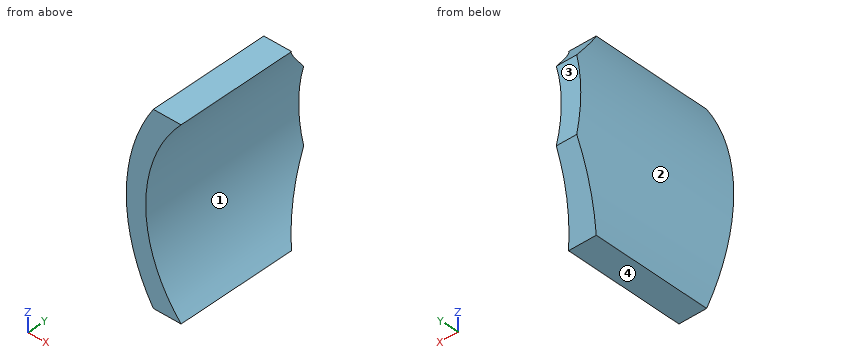
Autodesk Inventor part; units mm, degrees
ref_plane "YZ Plane" through (0, 0, 0) normal (1, 0, 0) x (0, 1, 0)
ref_plane "XZ Plane" through (0, 0, 0) normal (0, 1, 0) x (-1, 0, 0)
ref_plane "XY Plane" through (0, 0, 0) normal (0, 0, 1) x (1, 0, 0)
sketch "Sketch1" plane through (0, 0, 0) normal (0, 1, 0) x (-1, 0, 0)
  arc A0 (0, -7.5) -> (0, 7.5) centre (0, 0) ccw
  line L0 (0, 7.5) -> (0, -7.5)
  dimension "d0" = 15
extrude "Extrusion1" add sketch "Sketch1" along normal blind 12
ref_plane "Work Plane1" through (-10, 0, 7.5) normal (1, 0, 0) x (0, 0, -1)
sketch "Sketch2" plane through (-10, 0, 7.5) normal (1, 0, 0) x (0, 0, -1)
  line L0 (2.5, 8.0057) -> (2.5, 1.5057)
  line L1 (2.5, 1.5057) -> (12.5, 1.5057)
  line L2 (12.5, 1.5057) -> (12.5, 8)
  line L3 (9.5, 10.5) -> (5.5, 10.5)
  line L4 (9.5, 10.5) -> (12.5, 8)
  line L5 (5.5, 10.5) -> (2.5, 8.0057)
  line L6 (15, 0) -> (15, 12)
  point P0 (7.5, 0)
  dimension "d9" = 10
  dimension "d10" = 6.5
  dimension "d12" = 4
  dimension "d14" = 3
  dimension "d15" = 3
  dimension "d24" = 2.5
extrude "Extrusion2" add sketch "Sketch2" along normal blind 10
sketch "Sketch5" plane through (0, 0, 0) normal (0, 1, 0) x (-1, 0, 0)
  arc A0 (0, -7.5) -> (0, 7.5) centre (0, 0) ccw
  arc A1 (0, -7.5) -> (0, 7.5) centre (0, 0) ccw
  line L0 (0, 7.5) -> (0, -7.5)
  line L1 (0, -7.5) -> (0, 7.5)
extrude "Extrusion5" cut sketch "Sketch5" along normal through all both and the other way through all
sketch "Sketch6" plane through (0, 0, 0) normal (0, 1, 0) x (-1, 0, 0)
  line L0 (7.0902, 5) -> (5.5902, 5)
  arc A0 (7.0902, -5) -> (7.0902, 5) centre (12.3734, 0) ccw
  arc A1 (7.0902, -5) -> (7.0902, 5) centre (-0.7358, 0) ccw
  point P0 (0, 0)
extrude "Extrusion6" cut sketch "Sketch6" along normal through all both and the other way through all
properties part number "15mm_radius_mold_with_crystal_skull"
Work out the finished part from the listing and answer in its coordinate system (mm). Face numbers are marked on the shaded views. Coordinates: 2 decimals unless noted, no trailing zeros. Order: outer loops, then holes, each group sorted by start corner. A loop starts at its lowest first (then second) coordinate and runs counter-clockwise, first axis right, second up. Notation, with made-up numbers: (35.5, 62) - (44.5, 62) arc R13 ccw to (44.5, 74) - close; hole circle Ø7 at (89.25, -5.75). An arc over 180 degrees is marked (long way). Answer as a JSON object with one key per item and string values.
1. The mould has two halves that part along Z. Classify the marked faces 1, 2, 3 and 4: +Z half, -Z half, draft (parallel to the pull), parting line (faces both ways), or undercut.
Output values:
{"face 1": "undercut", "face 2": "parting line", "face 3": "draft", "face 4": "-Z half"}
2. Find section A-A on x = -6.2. Determine the outline of the cut face in (y, z), plus the area to 3 significant figures.
Output values:
{"outline": "(1.51, -5) - (8, -5) - (8.65, -4.22) - (1.51, -4.22) - close; (1.51, 4.22) - (8.65, 4.22) - (8.01, 5) - (1.51, 5) - close", "area": "10.6 mm²"}
3. Each of these flat-tipped pins is pushed along its axis until it touches: P1, Ø5, axis at y = 8, z = 0.5, coming from the +X side; P2, Ø1.5, axis at x = -6.5, y = 9, coming from the +Z side; P3, Ø3, axis at y = 3.5, z = 0.5, coming from the -X side. Where does it stop, or does it pass through?
Output values:
{"P1": "stops at x = -6.87", "P2": "stops at z = 4.71", "P3": "stops at x = -8.55"}
4. Consider line 1 (Z direction, x = -6.9, y = 7.25); line 2 (Z direction, x = -6.7, y = 6.75); line 3 (X direction, y = 6, z = 0). Determine where each line is inside the solid, lowest interval first.
Output values:
{"line 1": "z = -5 to -2.94, 2.94 to 5", "line 2": "z = -5 to -3.37, 3.37 to 5", "line 3": "x = -8.55 to -7.5"}
5. Find section D-D on z = 2.75. Determine the outline of the cut face in (x, y).
Output values:
{"outline": "(-8.13, 1.51) - (-6.98, 1.51) - (-6.98, 9.88) - (-8.13, 9.88) - close"}
6. Find section C-C on y = 3.25. Determine the outline of the cut face in (x, z), plus the area to 3 significant figures.
Output values:
{"outline": "(-7.09, -5) - (-5.59, -5) arc R7.5 cw to (-5.59, 5) - (-7.09, 5) arc R9.29 ccw to start", "area": "11.8 mm²"}
7. Find section B-B on x = -6.95. Determine the outline of the cut face in (y, z), plus the area to 3 significant figures.
Output values:
{"outline": "(1.51, -5) - (8, -5) - (9.82, -2.82) - (1.51, -2.82) - close; (1.51, 2.82) - (9.82, 2.82) - (8.01, 5) - (1.51, 5) - close", "area": "32.3 mm²"}
